```python
from build123d import *

# Parameters (mm, degrees)
SKETCH_1_R          = 6
EXTRUDE_1_DEPTH     = 30
SKETCH_2_R          = 3
EXTRUDE_2_DEPTH     = 12.5
SKETCH_4_R          = 2.5
CUT_EXTRUDE_1_DEPTH = 10


with BuildPart() as part:
    # 草图1 → 凸台-拉伸1 (new, symmetric)
    with BuildSketch(Plane.XY):
        Circle(SKETCH_1_R)
    extrude(amount=EXTRUDE_1_DEPTH, both=True)

    # 草图2 → 凸台-拉伸2 (add)
    with BuildSketch(Plane(origin=(0, 0, -30), x_dir=(-1, 0, 0), z_dir=(0, 0, -1))):
        with Locations(Location((0, 0, 0), (0, 0, 180))):
            Circle(SKETCH_2_R)
    extrude(amount=EXTRUDE_2_DEPTH)

    # 草图4 → 切除-拉伸1 (cut)
    with BuildSketch(Plane.XY.offset(30)):
        Circle(SKETCH_4_R)
    extrude(amount=-CUT_EXTRUDE_1_DEPTH, mode=Mode.SUBTRACT)


solid = part.part
```
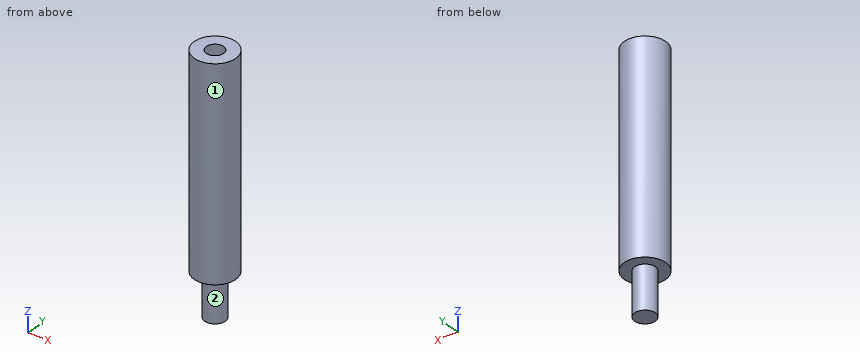
Could you check a few things on this model? Use its own coordinates, in mm. Face numbers are marked on the shaded views. A direction names the side the tool comes from. Round coordinates to 2 decimals unless told otherwise and drop trailing zeros. Loops run counter-clockwise (first coordinate to the right, second up) from the corner with the lowest first, then second, coordinate; pieces in that order, holes last. Notation, with made-up numbers: (-10, -1.75) - (45, -1.75) arc R20 cw to (45, 20.25) - close; hole circle Ø2 at (14, 62.5). An arc over 180 degrees is marked (long way). Answer as CSV lines item,"result".
1. For pin 1 Ø2 at (x, z) = (1.5, -6) entering from -Y; pin 2 Ø1 at (x, y) = (3.5, 3.5) entering from -Z; pin 3 Ø3 at (x, y) = (0, 0) entering from +Z, each with a flat end and sliding along its axis, tell me the tip position at first contact or that it passes through.
Filled in:
pin 1,"stops at y = -5.98"
pin 2,"stops at z = -30"
pin 3,"stops at z = 20"
2. I want a section at D-D on z = -22.5. List the corners of the cut face in (x, y) for me, then the cut area to 3 significant figures.
Filled in:
outline,"circle Ø12 at (0, 0)"
area,"113 mm^2"
3. I want a section at C-C on z = -32. List the corners of the cut face in (x, y) for me.
Filled in:
outline,"circle Ø6 at (0, 0)"
4. On a 3-axis mill with a long thin cutter (end or side, diameter ignored), from which of +Z, -Z, +X, -X, +Y, -Y can I reach the whole of each face in a straight line? I mean the marked faces 1 and 2. Say none if no direction works.
Filled in:
face 1,"+Z, -Z"
face 2,"-Z"
5. Please list where these lines run through material, in increasing order: line 1 along Y through (x, z) = (0, 22.5); line 2 along Z through (x, y) = (-4.5, 3); line 3 along Z through (x, y) = (-1, -0.75). Write a range as [from, to].
Filled in:
line 1,"y = [-6, -2.5], [2.5, 6]"
line 2,"z = [-30, 30]"
line 3,"z = [-42.5, 20]"
6. I want a section at A-A on y = 0. List the corners of the cut face in (x, z) for me, then the cut area to 3 significant figures.
Filled in:
outline,"(-6, -30) - (-3, -30) - (-3, -42.5) - (3, -42.5) - (3, -30) - (6, -30) - (6, 30) - (2.5, 30) - (2.5, 20) - (-2.5, 20) - (-2.5, 30) - (-6, 30) - close"
area,"745 mm^2"
